```python
from build123d import *

# Parameters (mm, degrees)
SKETCH1_R               = 6
BOSS_EXTRUDE1_DEPTH     = 7
SKETCH2_R               = 7.2
BOSS_EXTRUDE2_DEPTH     = 1.25
SKETCH3_R               = 7.2
BOSS_EXTRUDE3_DEPTH     = 1.25
SKETCH4_R               = 6
BOSS_EXTRUDE4_DEPTH     = 6
CUT_EXTRUDE2_DEPTH      = 19.836570813
CUT_EXTRUDE2_DEPTH_BACK = 11
SKETCH6_R               = 4
BOSS_EXTRUDE5_DEPTH     = 6


with BuildPart() as part:
    # Sketch1 → Boss-Extrude1 (new body)
    with BuildSketch(Plane(origin=(0, 0, 0), x_dir=(1, 0, 0), z_dir=(0, 1, 0))):
        with Locations(Location((0, 0.72, 0), (0, 0, 270))):
            Circle(SKETCH1_R)
    extrude(amount=BOSS_EXTRUDE1_DEPTH)

    # Sketch2 → Boss-Extrude2 (add)
    with BuildSketch(Plane(origin=(0, 7, 0), x_dir=(1, 0, 0), z_dir=(0, 1, 0))):
        with Locations(Location((0, 0.72, 0), (0, 0, 270))):
            Circle(SKETCH2_R)
    extrude(amount=BOSS_EXTRUDE2_DEPTH)

    # Sketch3 → Boss-Extrude3 (add)
    with BuildSketch(Plane(origin=(0, 8.25, 0), x_dir=(1, 0, 0), z_dir=(0, 1, 0))):
        with Locations(Location((0, -0.72, 0), (0, 0, 174.260829523))):
            Circle(SKETCH3_R)
    extrude(amount=BOSS_EXTRUDE3_DEPTH)

    # Sketch4 → Boss-Extrude4 (add)
    with BuildSketch(Plane(origin=(0, 9.5, 0), x_dir=(1, 0, 0), z_dir=(0, 1, 0))):
        with Locations(Location((0, -0.72, 0), (0, 0, 270))):
            Circle(SKETCH4_R)
    extrude(amount=BOSS_EXTRUDE4_DEPTH)

    # Sketch5 → Cut-Extrude2 (cut, two sides: drawn at the far end of the back side and taken through both)
    with BuildSketch(Plane.XZ.offset(-CUT_EXTRUDE2_DEPTH_BACK)):
        with BuildLine():
            Line((1.5, 2), (-1.5, 2))
            ThreePointArc((-1.5, 2), (0, -2.5), (1.5, 2))
        make_face()
    extrude(amount=CUT_EXTRUDE2_DEPTH + CUT_EXTRUDE2_DEPTH_BACK, mode=Mode.SUBTRACT)

    # Sketch6 → Boss-Extrude5 (add)
    with BuildSketch(Plane(origin=(0, 15.5, 0), x_dir=(1, 0, 0), z_dir=(0, 1, 0))):
        with Locations(Location((0, 0, 0), (0, 0, 270))):
            Circle(SKETCH6_R)
    extrude(amount=BOSS_EXTRUDE5_DEPTH)


solid = part.part
```
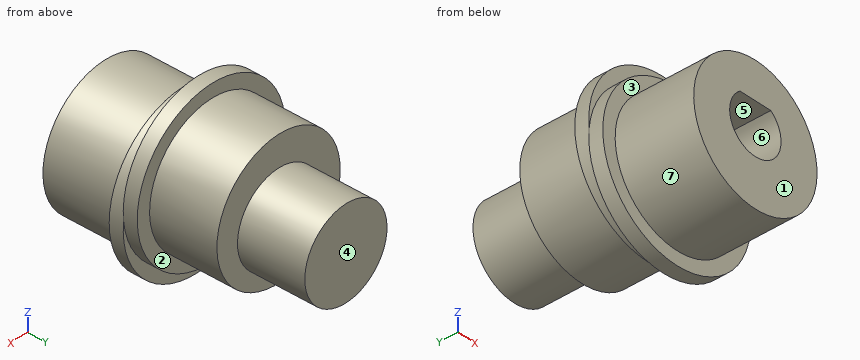
Verification items for the finished model (mm, model axes). Face numbers are marked on the shaded views. A direction names the side the tool comes from. Give positions to 0.01 mm unless a question says otherwise; leave off trailing zeros. Write each loop counter-clockwise with the first axis right and the second up, starting at its lowest first coordinate (ties: lowest second). Pieces come first, ordered by that corner, then holes. Notation, with made-up numbers: M -8.5,-1.75 L 25.5,-1.75 A21 ccw 25.5,13.25 Z; hole C 48,-32 d5. An arc over 180 degrees is marked long. One line per question, with ' | ' between items.
1) Section check C-C on y = 2.5. Enter the section's corners in (x, z).
Result:
outline: C 0,-0.72 d12; hole M -1.5,2 A2.5 ccw long 1.5,2 Z
2) Section check D-D on y = 12.25. Enter the section's corners in (x, z).
Result:
outline: C 0,0.72 d12
3) Gauge pin test, flat ends, axial feed: pin 1 Ø2 at (y, z) = (8.5, 2.5) entering from -X; pin 2 Ø1.5 at (x, y) = (5, 12) entering from +Z; pin 3 Ø5 at (x, y) = (2.5, 19) entering from +Z. Record the tip position at first contact, or that the pin passes through.
Result:
pin 1: stops at x = -7.16 | pin 2: stops at z = 4.96 | pin 3: stops at z = 4
4) Mould release check, pull along X, two halves, no side actions. Record for the marked faces 4, 5, 6 and 7: released by +X, released by -X, zero draft, split by the parting line, or undercut.
Result:
face 4: zero draft | face 5: undercut | face 6: undercut | face 7: split by the parting line
5) Set-up check for the marked faces 1, 2 and 3: record each of +Z, -Z, +X, -X, +Y, -Y from which the full face is reachable in a straight line by a thin tool's end or side.
Result:
face 1: +Z, -Z, +X, -X, -Y | face 2: +Y | face 3: -Y
6) Section check A-A on x = 0. Enter the section's corners in (y, z).
Result:
outline: M 0,-6.72 L 7,-6.72 L 7,-7.92 L 8.25,-7.92 L 8.25,-6.48 L 9.5,-6.48 L 9.5,-5.28 L 15.5,-5.28 L 15.5,-4 L 21.5,-4 L 21.5,4 L 15.5,4 L 15.5,6.72 L 9.5,6.72 L 9.5,7.92 L 8.25,7.92 L 8.25,6.48 L 7,6.48 L 7,5.28 L 0,5.28 L 0,2 L 11,2 L 11,-2.5 L 0,-2.5 Z
7) Section check B-B on z = 3. Enter the section's corners in (x, y).
Result:
outline: M -6.83,8.25 L -6.16,8.25 L -6.16,7 L -4.71,7 L -4.71,0 L 4.71,0 L 4.71,7 L 6.16,7 L 6.16,8.25 L 6.83,8.25 L 6.83,9.5 L 5.55,9.5 L 5.55,15.5 L 2.65,15.5 L 2.65,21.5 L -2.65,21.5 L -2.65,15.5 L -5.55,15.5 L -5.55,9.5 L -6.83,9.5 Z
8) Thickness scan on line 1 along Z through (x, y) = (0, 7.5); line 2 along Y through (x, z) = (1.5, 5); line 3 along Y through (x, z) = (-5.5, -4.25). Record the ranges inside material, lowest first. Write a range as [from, to].
Result:
line 1: z = [-7.92, -2.5], [2, 6.48] | line 2: y = [0, 15.5] | line 3: y = [7, 8.25]
